Geometry check sheet. Reference: the model listing, model coordinates, mm. A direction names the side the tool comes from. Coordinates: 2 decimals unless noted, no trailing zeros. Loops run counter-clockwise (first coordinate to the right, second up) from the corner with the lowest first, then second, coordinate; pieces in that order, holes last.
from build123d import *

# Parameters (mm, degrees)
F0_W     = 25
F0_H     = 25
F1_DEPTH = 25
F2_R     = 5
F3_T     = -3


# Not quite as in the source:
# - a shell that OpenCascade refuses in one call is made with other operations: the cavity is built on its own and cut out


with BuildPart() as f1:
    # F0 (on Top) → F1 (new body)
    with BuildSketch(Plane.XY):
        with Locations((12.5, 12.5)):
            Rectangle(F0_W, F0_H)
    extrude(amount=F1_DEPTH)

    # F2
    f2_edges = [f1.edges().sort_by_distance(p)[0] for p in [
        (12.5, 0, 0),
        (25, 0, 12.5),
        (12.5, 0, 25),
        (25, 25, 12.5),
        (25, 12.5, 0),
        (25, 12.5, 25),
        (0, 25, 12.5),
        (0, 0, 12.5),
        (0, 12.5, 0),
        (0, 12.5, 25),
        (12.5, 25, 0),
        (12.5, 25, 25),
    ]]
    fillet(f2_edges, radius=F2_R)

    # F3: a shell. OpenCascade refuses it in one call, so the cavity is built on its own and cut out:
    # the body offset inwards by the wall thickness, plus a prism from it out through each open face.
    f3_core = offset(f1.part, amount=F3_T, mode=Mode.PRIVATE)
    f3_exits = [f3_core.faces().sort_by_distance(p)[0] for p in [
        (12.5, 12.5, 3),
    ]]
    add(f3_core, mode=Mode.SUBTRACT)
    extrude(f3_exits, amount=-F3_T, mode=Mode.SUBTRACT)


solid = f1.part
(1) Sectioned sample at D-D on y = 4.5. Record the cut outline in (x, z).
Findings:
outline: (0.03, 5) arc R4.97 ccw to (5, 0.03) - (20, 0.03) arc R4.97 ccw to (24.97, 5) - (24.97, 20) arc R4.97 ccw to (20, 24.97) - (5, 24.97) arc R4.97 ccw to (0.03, 20) - close; hole (3.06, 5) arc R1.94 ccw to (5, 3.06) - (20, 3.06) arc R1.94 ccw to (21.94, 5) - (21.94, 20) arc R1.94 ccw to (20, 21.94) - (5, 21.94) arc R1.94 ccw to (3.06, 20) - close
(2) Gauge pin test, flat ends, axial feed: pin 1 Ø7.5 at (x, y) = (12.5, 15) entering from -Z; pin 2 Ø10 at (y, z) = (9.5, 3) entering from +X; pin 3 Ø3 at (x, y) = (22.5, 3.5) entering from -Z; pin 4 Ø2.5 at (x, z) = (13, 2) entering from -Y. Record the tip position at first contact, or that the pin passes through.
Findings:
pin 1: stops at z = 22
pin 2: stops at x = 25
pin 3: stops at z = 0.2
pin 4: stops at y = 0.32
(3) Scan lines: L1, parallel to Y at x = 5, z = 10.75; L2, parallel to Z at x = 19.75, y = 8.25. Record each from-to range of solid material in increasing order.
Findings:
L1: y = 0 to 3, 22 to 25
L2: z = 22 to 25
(4) Access from +Z, -Z, +X, -X, +Y, -Y to the whole of each face (thin tool, end or side, straight path). Record for faces 5 (the cylindrical face through (13, 1, 2)), 6 (the cylindrical face through (12.6, 21.43, 3.6)), 7 (the flat face through (20, 12, 2)).
Findings:
face 5: -Z, +X, -X, -Y
face 6: none
face 7: -Z
(5) Sectioned sample at A-A on z = 18.25. Record the cut outline in (x, y).
Findings:
outline: (0, 5) arc R5 ccw to (5, 0) - (20, 0) arc R5 ccw to (25, 5) - (25, 20) arc R5 ccw to (20, 25) - (5, 25) arc R5 ccw to (0, 20) - close; hole (3, 5) arc R2 ccw to (5, 3) - (20, 3) arc R2 ccw to (22, 5) - (22, 20) arc R2 ccw to (20, 22) - (5, 22) arc R2 ccw to (3, 20) - close
(6) Sectioned sample at B-B on y = 7.25. Record the cut outline in (x, z).
Findings:
outline: (0, 5) arc R5 ccw to (5, 0) - (5, 3) arc R2 cw to (3, 5) - (3, 20) arc R2 cw to (5, 22) - (20, 22) arc R2 cw to (22, 20) - (22, 5) arc R2 cw to (20, 3) - (20, 0) arc R5 ccw to (25, 5) - (25, 20) arc R5 ccw to (20, 25) - (5, 25) arc R5 ccw to (0, 20) - close
(7) Sectioned sample at C-C on x = 2. Record the cut outline in (y, z), and give its area (3 significant figures).
Findings:
outline: (1, 5) arc R4 ccw to (5, 1) - (20, 1) arc R4 ccw to (24, 5) - (24, 20) arc R4 ccw to (20, 24) - (5, 24) arc R4 ccw to (1, 20) - close
area: 515 mm2
(8) Draft check along Y on faces 1 (the cylindrical face through (1, 2, 13)), 2 (the flat face through (12, 13, 25)), 3 (the cylindrical face through (21.4, 3.57, 12.6)), 4 (the cylindrical face through (13, 24, 2)). Enter one of: +Y half, -Y half, draft (parallel to the pull), parting line (faces both ways), or undercut.
Findings:
face 1: -Y half
face 2: draft
face 3: undercut
face 4: +Y half
